Design review of the part built by this model. Coordinates are the model's own, in mm. A direction names the side the tool comes from. Coordinates: 2 decimals unless noted, no trailing zeros. Write each loop counter-clockwise with the first axis right and the second up, starting at its lowest first coordinate (ties: lowest second). Pieces come first, ordered by that corner, then holes. Notation, with made-up numbers: (55.25, 21) - (67.25, 21) arc R26 cw to (67.25, 37) - close; hole circle Ø7 at (65, 84). An arc over 180 degrees is marked (long way). Use a Markdown table: item, result.
from build123d import *

# Parameters (mm, degrees)
ESQUISSE1_W      = 105
ESQUISSE1_H      = 80
ESQUISSE1_R      = 1.5
EXTRUSION1_DEPTH = 3
ESQUISSE2_W      = 20
ESQUISSE2_H      = 20
ESQUISSE2_W_2    = 10
ESQUISSE2_H_2    = 10
EXTRUSION2_DEPTH = 3
ESQUISSE3_W      = 5
ESQUISSE3_H      = 10
ESQUISSE3_W_2    = 10
ESQUISSE3_H_2    = 5
EXTRUSION3_DEPTH = 15
ESQUISSE4_W      = 55
ESQUISSE4_H      = 5
EXTRUSION4_DEPTH = 5
ESQUISSE5_W      = 30
ESQUISSE5_H      = 20
EXTRUSION5_DEPTH = 3
ESQUISSE6_W      = 10
ESQUISSE6_H      = 7.5
EXTRUSION6_DEPTH = 5


with BuildPart() as part:
    # Esquisse1 → Extrusion1 (new body)
    with BuildSketch(Plane(origin=(0, 0, 0), x_dir=(1, 0, 0), z_dir=(0, 1, 0))):
        with Locations((52.5, 40)):
            Rectangle(ESQUISSE1_W, ESQUISSE1_H)
        with Locations((5, 75)):
            Circle(ESQUISSE1_R, mode=Mode.SUBTRACT)
        with Locations((100, 75)):
            Circle(ESQUISSE1_R, mode=Mode.SUBTRACT)
        with Locations((100, 5)):
            Circle(ESQUISSE1_R, mode=Mode.SUBTRACT)
        with Locations((5, 5)):
            Circle(ESQUISSE1_R, mode=Mode.SUBTRACT)
    extrude(amount=EXTRUSION1_DEPTH)

    # Esquisse2 → Extrusion2 (add)
    with BuildSketch(Plane(origin=(0, 3, 0), x_dir=(1, 0, 0), z_dir=(0, 1, 0))):
        with Locations((46.498714715, 59.553685436)):
            Rectangle(ESQUISSE2_W, ESQUISSE2_H)
        with Locations((44.830735419, 25.305948149)):
            Rectangle(ESQUISSE2_W_2, ESQUISSE2_H_2)
    extrude(amount=EXTRUSION2_DEPTH)

    # Esquisse3 → Extrusion3 (add)
    with BuildSketch(Plane(origin=(0, 3, 0), x_dir=(1, 0, 0), z_dir=(0, 1, 0))):
        with Locations((92.438953264, 61.221664733)):
            Rectangle(ESQUISSE3_W, ESQUISSE3_H)
        with Locations((14.058039322, 64.92274654)):
            Rectangle(ESQUISSE3_W_2, ESQUISSE3_H_2)
        with Locations((14.058039322, 54.92274654)):
            Rectangle(ESQUISSE3_W_2, ESQUISSE3_H_2)
        with Locations((14.058039322, 44.92274654)):
            Rectangle(ESQUISSE3_W_2, ESQUISSE3_H_2)
        with Locations((92.438953264, 41.221664733)):
            Rectangle(ESQUISSE3_W, ESQUISSE3_H)
        with Locations((92.438953264, 21.221664733)):
            Rectangle(ESQUISSE3_W, ESQUISSE3_H)
    extrude(amount=EXTRUSION3_DEPTH)

    # Esquisse4 → Extrusion4 (add)
    with BuildSketch(Plane.XZ):
        with Locations((62.5, -5)):
            Rectangle(ESQUISSE4_W, ESQUISSE4_H)
        with Locations((62.5, -75)):
            Rectangle(ESQUISSE4_W, ESQUISSE4_H)
    extrude(amount=EXTRUSION4_DEPTH)

    # Esquisse5 → Extrusion5 (add)
    with BuildSketch(Plane.XZ):
        with Locations((10, -23.761311795)):
            Rectangle(ESQUISSE5_W, ESQUISSE5_H)
    extrude(amount=EXTRUSION5_DEPTH)

    # Esquisse6 → Extrusion6 (add)
    with BuildSketch(Plane(origin=(0, 3, 0), x_dir=(1, 0, 0), z_dir=(0, 1, 0))):
        with Locations((105, 16.524993395)):
            Rectangle(ESQUISSE6_W, ESQUISSE6_H)
    extrude(amount=EXTRUSION6_DEPTH)


solid = part.part
(1) For pin 1 (8 mm diameter, centred on x = 105.5, z = -17, fed in from +Y); pin 2 (1.5 mm diameter, centred on x = 46, y = 5, fed in from +Z); pin 3 (2.5 mm diameter, centred on y = -3, z = -5, fed in from +X), all flat-tipped, find the tip position at first contact; note any pin that passes through.
Determined:
| item | result |
|---|---|
| pin 1 | y = 8 |
| pin 2 | z = -20.31 |
| pin 3 | x = 90 |
(2) Machinability: for faces 1 (the flat face through (89.939, 10, -61)), 2 (the flat face through (92, 10, -26.222)), 3 (the flat face through (14, 10, -47.423)), 4 (the flat face through (45, 6, -25)), 5 (the flat face through (10, -1, -13.761)), which of the approach directions +Z, -Z, +X, -X, +Y, -Y give a long, thin tool a straight path to every point of the face, cutting with its end or side? Answer none if there is none.
Determined:
| item | result |
|---|---|
| face 1 | +Z, -Z, +Y |
| face 2 | +X, +Y |
| face 3 | +X, -X, +Y |
| face 4 | +Z, -Z, -X, +Y |
| face 5 | +Z, +X, -X, -Y |
(3) Take a section at A-A on z = -5. Write out the cut boundary in (x, y).
Determined:
| item | result |
|---|---|
| outline | (0, 0) - (3.5, 0) - (3.5, 3) - (0, 3) - close; (6.5, 0) - (35, 0) - (35, -5) - (90, -5) - (90, 0) - (98.5, 0) - (98.5, 3) - (6.5, 3) - close; (101.5, 0) - (105, 0) - (105, 3) - (101.5, 3) - close |
(4) Take a section at B-B on y = 13. Write out the cut boundary in (x, z).
Determined:
| item | result |
|---|---|
| outline | (9.06, -67.42) - (19.06, -67.42) - (19.06, -62.42) - (9.06, -62.42) - close; (9.06, -57.42) - (19.06, -57.42) - (19.06, -52.42) - (9.06, -52.42) - close; (9.06, -47.42) - (19.06, -47.42) - (19.06, -42.42) - (9.06, -42.42) - close; (89.94, -66.22) - (94.94, -66.22) - (94.94, -56.22) - (89.94, -56.22) - close; (89.94, -46.22) - (94.94, -46.22) - (94.94, -36.22) - (89.94, -36.22) - close; (89.94, -26.22) - (94.94, -26.22) - (94.94, -16.22) - (89.94, -16.22) - close |
(5) For L1, parallel to Z at x = 5, y = 1.8; L2, parallel to X at y = 0.85, z = -75; L3, parallel to X at y = 6, z = -19, list the stretches that pass through material, from the lowest coordinate up. Write a range as from..to.
Determined:
| item | result |
|---|---|
| L1 | -80..-76.5, -73.5..-6.5, -3.5..0 |
| L2 | 0..3.5, 6.5..98.5, 101.5..105 |
| L3 | 89.94..94.94, 100..110 |
(6) Draft analysis for pull direction Z (two halves, no side actions). For faces 6 (the flat face through (92, 10, -16.222)), 7 (the flat face through (14, 10, -57.423)), 8 (the flat face through (25, -1, -24)), state which applies: +Z half, -Z half, draft (parallel to the pull), parting line (faces both ways), or undercut.
Determined:
| item | result |
|---|---|
| face 6 | +Z half |
| face 7 | undercut |
| face 8 | draft |
(7) Take a section at D-D on x = 5. Write out the cut boundary in (y, z).
Determined:
| item | result |
|---|---|
| outline | (-3, -33.76) - (0, -33.76) - (0, -73.5) - (3, -73.5) - (3, -6.5) - (0, -6.5) - (0, -13.76) - (-3, -13.76) - close; (0, -80) - (3, -80) - (3, -76.5) - (0, -76.5) - close; (0, -3.5) - (3, -3.5) - (3, 0) - (0, 0) - close |
(8) Take a section at C-C on x = 53.5. Write out the cut boundary in (y, z).
Determined:
| item | result |
|---|---|
| outline | (-5, -77.5) - (0, -77.5) - (0, -80) - (3, -80) - (3, -69.55) - (6, -69.55) - (6, -49.55) - (3, -49.55) - (3, 0) - (0, 0) - (0, -2.5) - (-5, -2.5) - (-5, -7.5) - (0, -7.5) - (0, -72.5) - (-5, -72.5) - close |
